Work out the finished part from the listing and answer in its coordinate system (mm). Give positions to 0.01 mm unless a question says otherwise; leave off trailing zeros. Order: outer loops, then holes, each group sorted by start corner. A loop starts at its lowest first (then second) coordinate and runs counter-clockwise, first axis right, second up. Notation, with made-up numbers: (77, 42) - (110, 42) arc R19 cw to (110, 68) - close; hole circle Ø8 at (-19.5, 85.25). An arc over 180 degrees is marked (long way). Put each result on its own line as item: value.
```python
from build123d import *

# Parameters (mm, degrees)
SKICA1_W                 = 191
SKICA1_H                 = 285
P_IDAT_VYSUNUT_M1_DEPTH  = 3
SKICA7_W                 = 25
SKICA7_H                 = 3
P_IDAT_VYSUNUT_M2_DEPTH  = 3
SKICA6_W                 = 3
SKICA6_H                 = 5
ODEBRAT_VYSUNUT_M6_DEPTH = 175.067515637
SKICA4_W                 = 3
SKICA4_H                 = 25
ODEBRAT_VYSUNUT_M3_DEPTH = 175.067515637


with BuildPart() as part:
    # Skica1 → Přidat vysunutím1 (new body)
    with BuildSketch(Plane(origin=(0, 0, 0), x_dir=(1, 0, 0), z_dir=(0, 1, 0))):
        Rectangle(SKICA1_W, SKICA1_H)
    extrude(amount=P_IDAT_VYSUNUT_M1_DEPTH)

    # Skica7 → Přidat vysunutím2 (add)
    with BuildSketch(Plane(origin=(0, 0, 0), x_dir=(1, 0, 0), z_dir=(0, 1, 0))):
        with Locations((-75, -144)):
            Rectangle(SKICA7_W, SKICA7_H)
        with Locations((-25, -144)):
            Rectangle(SKICA7_W, SKICA7_H)
        with Locations((25, -144)):
            Rectangle(SKICA7_W, SKICA7_H)
        with Locations((75, -144)):
            Rectangle(SKICA7_W, SKICA7_H)
        with Locations((75, 144)):
            Rectangle(SKICA7_W, SKICA7_H)
        with Locations((25, 144)):
            Rectangle(SKICA7_W, SKICA7_H)
        with Locations((-25, 144)):
            Rectangle(SKICA7_W, SKICA7_H)
        with Locations((-75, 144)):
            Rectangle(SKICA7_W, SKICA7_H)
    extrude(amount=P_IDAT_VYSUNUT_M2_DEPTH)

    # Skica6 → Odebrat vysunutím6 (cut, through all)
    with BuildSketch(Plane(origin=(0, 0, 0), x_dir=(1, 0, 0), z_dir=(0, 1, 0))):
        with Locations((-90, -135)):
            Rectangle(SKICA6_W, SKICA6_H)
        with Locations((90, -135)):
            Rectangle(SKICA6_W, SKICA6_H)
        with Locations((90, 135)):
            Rectangle(SKICA6_W, SKICA6_H)
        with Locations((-90, 135)):
            Rectangle(SKICA6_W, SKICA6_H)
    extrude(amount=ODEBRAT_VYSUNUT_M6_DEPTH, mode=Mode.SUBTRACT)

    # Skica4 → Odebrat vysunutím3 (cut, through all)
    with BuildSketch(Plane(origin=(0, 0, 0), x_dir=(1, 0, 0), z_dir=(0, 1, 0))):
        with Locations((-66.5, 110)):
            Rectangle(SKICA4_W, SKICA4_H)
        with Locations((0, 110)):
            Rectangle(SKICA4_W, SKICA4_H)
        with Locations((66.5, 110)):
            Rectangle(SKICA4_W, SKICA4_H)
        with Locations((66.5, 60)):
            Rectangle(SKICA4_W, SKICA4_H)
        with Locations((0, 60)):
            Rectangle(SKICA4_W, SKICA4_H)
        with Locations((-66.5, 60)):
            Rectangle(SKICA4_W, SKICA4_H)
        with Locations((66.5, 10)):
            Rectangle(SKICA4_W, SKICA4_H)
        with Locations((0, 10)):
            Rectangle(SKICA4_W, SKICA4_H)
        with Locations((-66.5, 10)):
            Rectangle(SKICA4_W, SKICA4_H)
        with Locations((66.5, -40)):
            Rectangle(SKICA4_W, SKICA4_H)
        with Locations((0, -40)):
            Rectangle(SKICA4_W, SKICA4_H)
        with Locations((-66.5, -40)):
            Rectangle(SKICA4_W, SKICA4_H)
        with Locations((66.5, -90)):
            Rectangle(SKICA4_W, SKICA4_H)
        with Locations((0, -90)):
            Rectangle(SKICA4_W, SKICA4_H)
        with Locations((-66.5, -90)):
            Rectangle(SKICA4_W, SKICA4_H)
    extrude(amount=ODEBRAT_VYSUNUT_M3_DEPTH, mode=Mode.SUBTRACT)


solid = part.part
```
(1) Given pin 1 (1.5 mm diameter, centred on y = 1, z = -144, fed in from +X); pin 2 (1.5 mm diameter, centred on x = 0, y = 2, fed in from +Z), each flat-ended and moving along its own axis, determine where each tip first touches the part or whether it passes through.
Geometry check:
pin 1: stops at x = 87.5
pin 2: stops at z = 142.5
(2) Section B-B, the plane y = 2.05 is taken. Count the separate pieces of the cut face and the enclosed holes in it, then the cut area to 4 significant figures.
Geometry check:
separate pieces: 1
enclosed holes: 19
area: 53,850 mm²
(3) Straight lines are drawn through the part: line 1 (X direction, y = 2.5, z = 36); line 2 (Z direction, x = -1, y = 1); line 3 (Z direction, x = 48, y = 0.9). For each, find the intervals that lie inside material, in ascending order.
Geometry check:
line 1: x = -95.5 to -68, -65 to -1.5, 1.5 to 65, 68 to 95.5
line 2: z = -142.5 to -122.5, -97.5 to -72.5, -47.5 to -22.5, 2.5 to 27.5, 52.5 to 77.5, 102.5 to 142.5
line 3: z = -142.5 to 142.5
(4) Section A-A, the plane z = -52 is taken. Write down the section's boundary in (x, y).
Geometry check:
outline: (-95.5, 0) - (-68, 0) - (-68, 3) - (-95.5, 3) - close; (-65, 0) - (-1.5, 0) - (-1.5, 3) - (-65, 3) - close; (1.5, 0) - (65, 0) - (65, 3) - (1.5, 3) - close; (68, 0) - (95.5, 0) - (95.5, 3) - (68, 3) - close
(5) Section C-C, the plane x = 42 is taken. Write down the section's boundary in (y, z).
Geometry check:
outline: (0, -142.5) - (3, -142.5) - (3, 142.5) - (0, 142.5) - close
